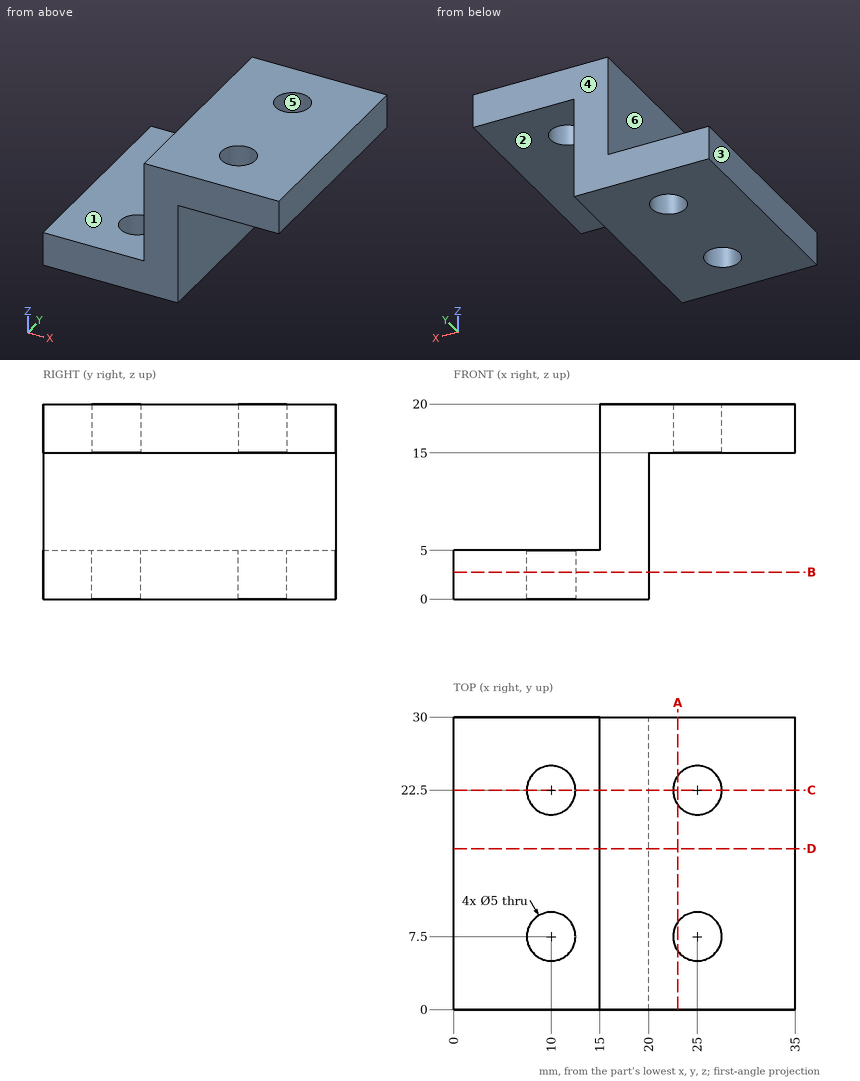
The drawing under review shows one solid part. Ordinate dimensions are in mm from its lowest x, y, z. A direction names the side the tool comes from. Give positions to 0.01 mm unless a question says otherwise; leave off trailing zeros. Order: outer loops, then holes, each group sorted by start corner. A loop starts at its lowest first (then second) coordinate and runs counter-clockwise, first axis right, second up. Notation, with made-up numbers: (-29, 54.5) -> (14, 54.5) arc R7 cw to (14, 62.5) -> close; hole circle Ø5 at (52, 55). An arc over 180 degrees is marked (long way). Write item = value, one per line. Start each with the question number.
(1) We need section A-A on x = 23. Write out the cut boundary in (y, z), plus the area to 3 significant figures.
(2) We need section C-C on y = 22.5. Write out the cut boundary in (x, z), plus the area to 3 significant figures.
(3) Mouldability with a two-part tool opening along Y and no side actions: class the marked faces 4, 5 and 6 as +Y half, -Y half, draft (parallel to the pull), parting line (faces both ways), or undercut.
(4) For pin 1 (4.5 mm diameter, centred on y = 11, z = 11, fed in from +X); pin 2 (7.5 mm diameter, centred on x = 24, y = 8, fed in from -Z); pin 3 (6 mm diameter, centred on x = 10, y = 22.5, fed in from +Z); pin 4 (4.5 mm diameter, centred on x = 25, y = 22.5, fed in from +Z), all flat-tipped, find the tip position at first contact; note any pin that passes through.
(5) For the marked faces 1, 2 and 3, list the 3-axis set-ups (+Z, -Z, +X, -X, +Y, -Y) from which the entire face can be reached by the end or side of a thin tool; tool diameter is ignored.
(6) To check wall thickness, follow line 1 along Y through (x, z) = (10, 2.3); line 2 along X through (y, z) = (9, 12.75); line 3 along Z through (x, y) = (4.5, 11). State the ranges of each line that lie inside material, in increasing order.
(7) We need section B-B on z = 2.75. Write out the cut boundary in (x, y).
(8) We need section D-D on y = 16.5. Write out the cut boundary in (x, z), plus the area to 3 significant figures.
Numbers:
q1.outline = (0, 15) -> (6, 15) -> (6, 20) -> (0, 20) -> close; (9, 15) -> (21, 15) -> (21, 20) -> (9, 20) -> close; (24, 15) -> (30, 15) -> (30, 20) -> (24, 20) -> close
q1.area = 120 mm^2
q2.outline = (0, 0) -> (7.5, 0) -> (7.5, 5) -> (0, 5) -> close; (12.5, 0) -> (20, 0) -> (20, 15) -> (22.5, 15) -> (22.5, 20) -> (15, 20) -> (15, 5) -> (12.5, 5) -> close; (27.5, 15) -> (35, 15) -> (35, 20) -> (27.5, 20) -> close
q2.area = 200 mm^2
q3.face_4 = +Y half
q3.face_5 = undercut
q3.face_6 = draft
q4.pin_1 = 20
q4.pin_2 = 15
q4.pin_3 = 5
q4.pin_4 = through
q5.face_1 = +Z, -X, +Y, -Y
q5.face_2 = -Z, +X, +Y, -Y
q5.face_3 = +Z, -Z, -X, +Y, -Y
q6.line_1 = 0 to 5, 10 to 20, 25 to 30
q6.line_2 = 15 to 20
q6.line_3 = 0 to 5
q7.outline = (0, 0) -> (20, 0) -> (20, 30) -> (0, 30) -> close; hole circle Ø5 at (10, 7.5); hole circle Ø5 at (10, 22.5)
q8.outline = (0, 0) -> (20, 0) -> (20, 15) -> (35, 15) -> (35, 20) -> (15, 20) -> (15, 5) -> (0, 5) -> close
q8.area = 250 mm^2
